Input: dimensioned drawing with shaded views. Units: mm. Origin: part minimum x, y, z. A direction names the side the tool comes from. Give positions to 0.01 mm unless a question says otherwise; leave off trailing zeros. Loops run counter-clockwise (first coordinate to the right, second up) from the corner with the lowest first, then second, coordinate; pieces in that order, holes last. Notation, with made-up numbers: (51, 41.5) -> (70, 41.5) arc R18 cw to (70, 58.5) -> close; hole circle Ø9 at (9, -4.5). An arc over 180 degrees is marked (long way). Answer in a Markdown table with one row per item. Add a question column.
1) Section query A-A (y = 20). Return the cut outline in (x, z).
2) Section query C-C (x = 64). Return the cut outline in (y, z), plus the area to 3 significant figures.
3) Access query for the marked faces 1, 2 and 3. Directions: +Z, -Z, +X, -X, +Y, -Y. A direction counts if a zero-diameter tool reaches every point of the face in a straight line with its end or side. Return the directions, or none.
4) First-contact query: P1, Ø12, axis at y = 11, z = 18.5, coming from the -X side; P2, Ø1, axis at y = 23.5, z = 33, coming from the -X side; P3, Ø6, axis at x = 48.5, z = 10.5, coming from the -Y side; P4, Ø2, axis at x = 78.5, y = 19, coming from the +Z side. Flat tips, straight axial feed; report the tip coordinate or a pass-through.
5) Section query D-D (z = 32). Return the cut outline in (x, y), plus the area to 3 significant figures.
6) Line query: line 1 (X direction, y = 3.5, z = 21.5); line 2 (Y direction, x = 42, z = 35); line 3 (Z direction, x = 46, y = 34). Output: solid intervals per line, ascending. Write a range as from..to.
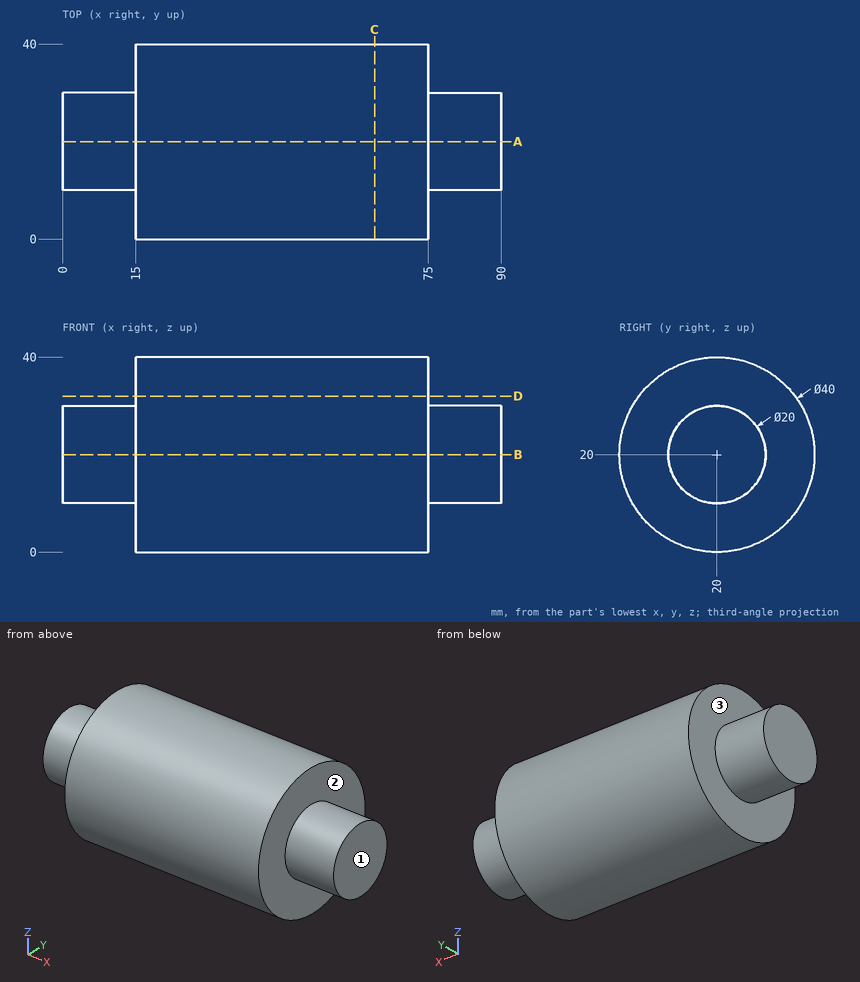
Evaluation:
| question | item | result |
|---|---|---|
| 1 | outline | (0, 10) -> (15, 10) -> (15, 0) -> (75, 0) -> (75, 10) -> (90, 10) -> (90, 30) -> (75, 30) -> (75, 40) -> (15, 40) -> (15, 30) -> (0, 30) -> close |
| 2 | outline | circle Ø40 at (20, 20) |
| 2 | area | 1,260 mm² |
| 3 | face 1 | +Z, -Z, +X, +Y, -Y |
| 3 | face 2 | +X |
| 3 | face 3 | -X |
| 4 | P1 | x = 0 |
| 4 | P2 | x = 15 |
| 4 | P3 | y = 1.09 |
| 4 | P4 | z = 30 |
| 5 | outline | (15, 4) -> (75, 4) -> (75, 36) -> (15, 36) -> close |
| 5 | area | 1,920 mm² |
| 6 | line 1 | 15..75 |
| 6 | line 2 | 6.77..33.23 |
| 6 | line 3 | 5.72..34.28 |
